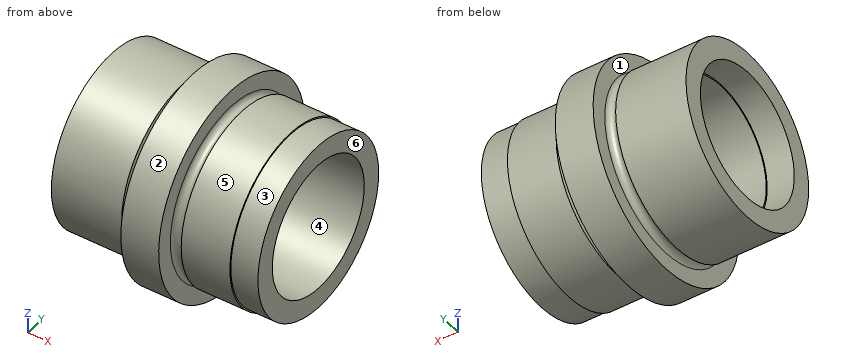
```python
from build123d import *


with BuildPart() as part:
    # Esboço1 → Revolução1 (revolve)
    with BuildSketch(Plane.XY, mode=Mode.PRIVATE) as revolu_o1_sk:
        with BuildLine():
            Line((0, 12.25), (0, 16))
            Line((0, 16), (13, 16))
            ThreePointArc((13, 16), (14, 15), (15, 16))
            Line((15, 16), (15, 19.05))
            Line((15, 19.05), (22, 19.05))
            Line((22, 19.05), (22, 16))
            ThreePointArc((22, 16), (23, 15), (24, 16))
            Line((24, 16), (33, 16))
            Line((33, 16), (33, 15.75))
            Line((33, 15.75), (38, 15.75))
            Line((38, 15.75), (38, 12))
            Line((38, 12), (5, 12))
            Line((5, 12), (5, 12.25))
            Line((5, 12.25), (0, 12.25))
        make_face()
    revolve(revolu_o1_sk.sketch.rotate(Axis((-90.616216216, 0, 0), (1, 0, 0)), 90), axis=Axis((-90.616216216, 0, 0), (1, 0, 0)))  # turned: the seam where the file's is


solid = part.part
```
Verification items for the finished model (mm, model axes). Face numbers are marked on the shaded views. A direction names the side the tool comes from. Round coordinates to 2 decimals unless told otherwise and drop trailing zeros. Write each loop counter-clockwise with the first axis right and the second up, starting at its lowest first coordinate (ties: lowest second). Pieces come first, ordered by that corner, then holes. Notation, with made-up numbers: (-1, -28) -> (41, -28) arc R25 ccw to (41, -9) -> close; hole circle Ø10 at (-39.5, -16.5). An arc over 180 degrees is marked (long way). Write each question's results on one line, items separated by ' | '. Start each with the question number.
1. Cross-section at C-C (x = 35). Enter the section's corners in (y, z).
2. Cross-section at A-A (y = 0). Enter the section's corners in (x, z).
3. Depth check by flat-ended pin: P1, Ø2, axis at x = 28.5, z = -8, coming from the +Y side; P2, Ø14.5, axis at y = 0, z = 0, coming from the -X side; P3, Ø4, axis at x = 14, y = -13.5, coming from the +Z side; P4, Ø12, axis at x = 28.5, y = -3.5, coming from the +Z side. Enter the tip coordinate at first touch or a pass-through.
4. Set-up check for the marked faces 1, 2 and 3: record each of +Z, -Z, +X, -X, +Y, -Y from which the full face is reachable in a straight line by a thin tool's end or side.
5. Material ranges on probe 1 along Y at (x, z) = (4, 0); probe 2 along X at (y, z) = (-13, 8); probe 3 along Y at (x, z) = (27, 4), recorded low to high. Write a range as from..to.
6. Draft check along Z on the marked faces 4, 5 and 6. Enter one of: +Z half, -Z half, draft (parallel to the pull), parting line (faces both ways), or undercut.
Solutions:
1) outline: circle Ø31.5 at (0, 0); hole circle Ø24 at (0, 0)
2) outline: (0, -16) -> (13, -16) arc R1 cw to (15, -16) -> (15, -19.05) -> (22, -19.05) -> (22, -16) arc R1 cw to (24, -16) -> (33, -16) -> (33, -15.75) -> (38, -15.75) -> (38, -12) -> (5, -12) -> (5, -12.25) -> (0, -12.25) -> close; (0, 12.25) -> (5, 12.25) -> (5, 12) -> (38, 12) -> (38, 15.75) -> (33, 15.75) -> (33, 16) -> (24, 16) arc R1 cw to (22, 16) -> (22, 19.05) -> (15, 19.05) -> (15, 16) arc R1 cw to (13, 16) -> (0, 16) -> close
3) P1: stops at y = 14.39 | P2: passes through | P3: stops at z = 14.98 | P4: stops at z = 16
4) face 1: -X | face 2: +X, -X | face 3: +X
5) probe 1: y = -16..-12.25, 12.25..16 | probe 2: x = 0..13.32, 14.68..22.32, 23.68..38 | probe 3: y = -15.49..-11.31, 11.31..15.49
6) face 4: undercut | face 5: parting line | face 6: draft
